Autodesk Inventor part; units mm, degrees
ref_plane "YZ Plane" through (0, 0, 0) normal (1, 0, 0) x (0, 1, 0)
ref_plane "XZ Plane" through (0, 0, 0) normal (0, 1, 0) x (-1, 0, 0)
ref_plane "XY Plane" through (0, 0, 0) normal (0, 0, 1) x (1, 0, 0)
sketch "Szkic1" plane through (0, 0, 0) normal (0, 0, 1) x (1, 0, 0)
  line L0 (-7.5, -7.5) -> (7.5, -7.5)
  line L1 (7.5, -7.5) -> (7.5, 7.5)
  line L2 (7.5, 7.5) -> (-7.5, 7.5)
  line L3 (-7.5, 7.5) -> (-7.5, -7.5)
  line L4 (-7.5, -7.5) -> (7.5, 7.5) construction
  line L5 (7.5, -7.5) -> (-7.5, 7.5) construction
  line L6 (7.5, 7.5) -> (2.5, 7.5) construction
  line L7 (2.5, 7.5) -> (2.5, 3.5) construction
  line L8 (2.5, 3.5) -> (7.5, 3.5) construction
  line L9 (7.5, 3.5) -> (7.5, 7.5) construction
  line L10 (2.5, 6.8486) -> (5.4, 5.1743)
  line L11 (5.4, 5.1743) -> (5.4, 1.8257)
  line L12 (5.4, 1.8257) -> (2.5, 0.1514)
  line L13 (2.5, 0.1514) -> (-0.4, 1.8257)
  line L14 (-0.4, 1.8257) -> (-0.4, 5.1743)
  line L15 (-0.4, 5.1743) -> (2.5, 6.8486)
  point P0 (0, 0)
  dimension "d0" = 15
  dimension "d1" = 15
  dimension "d4" = 5
  dimension "d5" = 4
  dimension "d8" = 5.8
extrude "Wyciągnięcie proste1" add sketch "Szkic1" along normal blind 10 contours L3 L2 L1 L0 | L10 L11 L12 L13 L14 L15
sketch "Szkic2" plane through (7.5, -7.5, 0) normal (1, 0, 0) x (0, 0, -1)
  line L0 (0, 0) -> (-4, 0) construction
  line L1 (-4, 0) -> (-4, 5) construction
  line L2 (-4, 5) -> (0, 5) construction
  line L3 (0, 5) -> (0, 0) construction
  point P0 (0, 7.5)
  dimension "d6" = 4
  dimension "d7" = 5
hole "Otwór1" at (2.5, 3.5, 0) direction (0, 0, 1) diameter 3.5 end through all
extrude "Wyciągnięcie proste2" cut sketch "Szkic1" along normal blind 3 contours L10 L11 L12 L13 L14 L15
hole "Otwór2" at (7.5, -2.5, 4) direction (-1, 0, 0) diameter 3.5 end through all
sketch "Szkic3" plane through (0, 0, 10) normal (0, 0, 1) x (1, 0, 0)
  circle A0 centre (2.5, 3.5) radius 1.75
  line L0 (-0.4, 5.1743) -> (-0.4, 1.8257)
  line L1 (2.5, 6.8486) -> (-0.4, 5.1743)
  line L2 (2.5, 6.8486) -> (5.4, 5.1743)
  line L3 (5.4, 1.8257) -> (5.4, 5.1743)
  line L4 (2.5, 0.1514) -> (5.4, 1.8257)
  line L5 (2.5, 0.1514) -> (-0.4, 1.8257)
  point P0 (0, 0)
extrude "Wyciągnięcie proste3" cut sketch "Szkic3" against normal blind 2
fillet "Zaokrąglenie1" radius 2 5 edges at (-7.5, 7.5, 5) (-7.5, -7.5, 5) (-7.5, 0, 10) (0, 7.5, 10) (0, -7.5, 10)
sketch "Szkic4" plane through (0, 0, 3) normal (0, 0, -1) x (-1, 0, 0)
  circle A0 centre (-2.5, 3.5) radius 1.75
  point P0 (0, 0)
extrude "Wyciągnięcie proste4" add sketch "Szkic4" against normal blind 0.5
properties part number "Z_endstop_regulator"
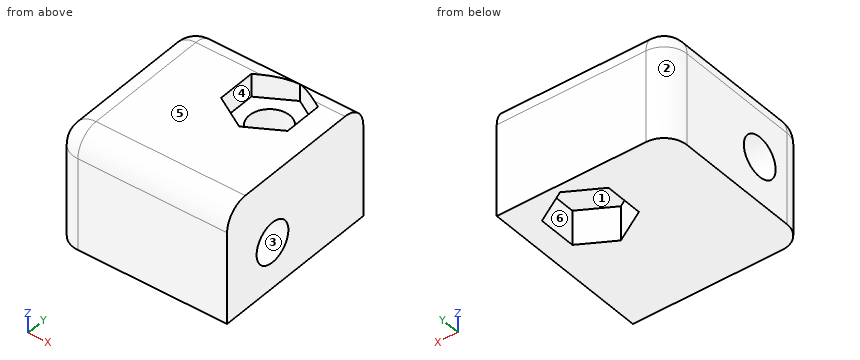
Part model, mm, in its own coordinate system. Face numbers are marked on the shaded views. A direction names the side the tool comes from. Give positions to 0.01 mm unless a question says otherwise; leave off trailing zeros. Write each loop counter-clockwise with the first axis right and the second up, starting at its lowest first coordinate (ties: lowest second). Pieces come first, ordered by that corner, then holes.
1) Cut at B-B on y = -2.5. Write the cut outline in (x, z).
Resolved:
outline: (-7.5, 0) - (7.5, 0) - (7.5, 2.25) - (-7.5, 2.25) - close; (-7.5, 5.75) - (7.5, 5.75) - (7.5, 10) - (-5.5, 10) arc R2 ccw to (-7.5, 8) - close
2) Probe L1, parallel to X at y = 3.5, z = 5.6; L2, parallel to Z at x = -2.5, y = -2.5; L3, parallel to Y at x = -2.5, z = 4. List the from-to ranges inside material, lowest first.
Resolved:
L1: x = -7.5 to 0.75, 4.25 to 7.5
L2: z = 0 to 2.25, 5.75 to 10
L3: y = -7.5 to -4.25, -0.75 to 7.5
3) Which spindle directions (+Z, -Z, +X, -X, +Y, -Y) get a long thin tool onto all of the face, cutting with end or side? Do the marked faces 4, 5 and 6. Say none if no direction does.
Resolved:
face 4: +Z
face 5: +Z, +X, -X, +Y, -Y
face 6: -Z
4) Cut at A-A on z = 4. Write the cut outline in (x, y), then the cut area to 3 significant figures.
Resolved:
outline: (-7.5, -5.5) arc R2 ccw to (-5.5, -7.5) - (7.5, -7.5) - (7.5, -4.25) - (-7.5, -4.25) - close; (-7.5, -0.75) - (7.5, -0.75) - (7.5, 7.5) - (-5.5, 7.5) arc R2 ccw to (-7.5, 5.5) - close; hole circle Ø3.5 at (2.5, 3.5)
area: 161 mm2
5) Two-plate mould, pull along X, no slides. Class the marked faces 1, 2 and 3: released by +X, released by -X, zero draft, split by the parting line, or undercut.
Resolved:
face 1: undercut
face 2: released by -X
face 3: zero draft
6) Cut at D-D on y = 3.5. Write the cut outline in (x, z), then the cut area to 3 significant figures.
Resolved:
outline: (-7.5, 0) - (-0.4, 0) - (-0.4, 3) - (5.4, 3) - (5.4, 0) - (7.5, 0) - (7.5, 10) - (5.4, 10) - (5.4, 8) - (4.25, 8) - (4.25, 3.5) - (0.75, 3.5) - (0.75, 8) - (-0.4, 8) - (-0.4, 10) - (-5.5, 10) arc R2 ccw to (-7.5, 8) - close
area: 104 mm2
7) Pin check, flat tips, straight feed: pin 1 (1 mm diameter, centred on x = 2, y = 3.5, fed in from +Z); pin 2 (3 mm diameter, centred on y = -2.5, z = 4, fed in from -X); pin 3 (1.7 mm diameter, centred on x = 1.5, y = 3.5, fed in from +Z). Stop position of each tip, or through.
Resolved:
pin 1: stops at z = 3.5
pin 2: passes through
pin 3: stops at z = 8
8) Cut at C-C on x = -3.5. Write the cut outline in (y, z), then the cut area to 3 significant figures.
Resolved:
outline: (-7.5, 0) - (7.5, 0) - (7.5, 8) arc R2 ccw to (5.5, 10) - (-5.5, 10) arc R2 ccw to (-7.5, 8) - close; hole circle Ø3.5 at (-2.5, 4)
area: 139 mm2
